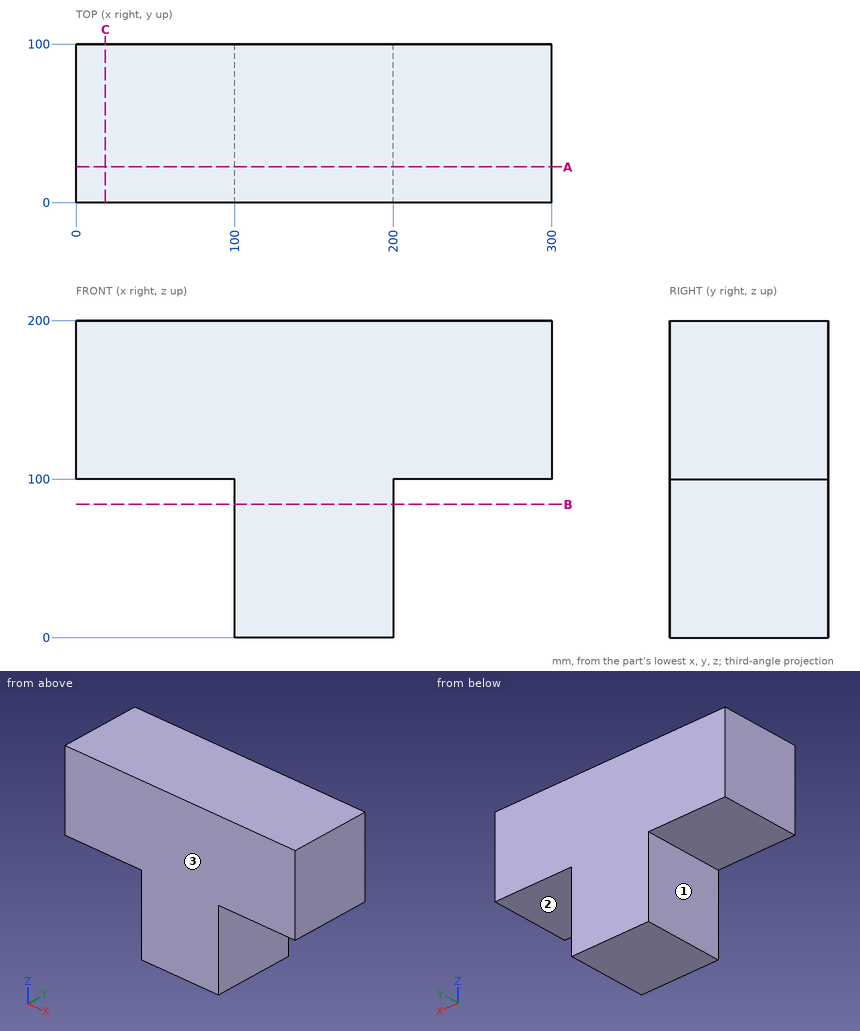
Study the drawing (mm; zero at the part's minimum x, y, z) and answer. A direction names the side the tool comes from. Give positions to 0.01 mm unless a question says otherwise; leave off trailing zeros. Order: outer loops, then holes, each group sorted by start corner. A loop starts at its lowest first (then second) coordinate and runs counter-clockwise, first axis right, second up. Notation, with made-up numbers: (-33.75, 50.25) -> (-11.75, 50.25) arc R21 ccw to (-11.75, 87.25) -> close; hole circle Ø2 at (-28.5, 19). An arc over 180 degrees is marked (long way). Put each result on its own line as item: value.
Item 1: For the marked faces 1, 2 and 3, determine the directions among +Z, -Z, +X, -X, +Y, -Y from which every point of the face is accessible in a straight line to the end or side of a thin tool.
Established:
face 1: -Z, -X, +Y, -Y
face 2: -Z, +X, +Y, -Y
face 3: +Z, -Z, +X, -X, -Y
Item 2: A straight line is drawn through the part: line 1 (Z direction, x = 80.5, y = 58.5). Find the intervals that lie inside material, in ascending order.
Established:
line 1: z = 100 to 200
Item 3: Given P1, Ø4, axis at y = 46.5, z = 130, coming from the -X side; P2, Ø1, axis at y = 37.5, z = 51, coming from the +X side; P3, Ø10, axis at x = 57.5, y = 60, coming from the -Z side, each flat-ended and moving along its own axis, determine where each tip first touches the part or whether it passes through.
Established:
P1: stops at x = 0
P2: stops at x = 200
P3: stops at z = 100
Item 4: A cutting plane is placed at A-A on y = 22.5. Give the vertices of the cut face in (x, z), plus the area to 3 significant figures.
Established:
outline: (0, 100) -> (100, 100) -> (100, 0) -> (200, 0) -> (200, 100) -> (300, 100) -> (300, 200) -> (0, 200) -> close
area: 40,000 mm^2
Item 5: A cutting plane is placed at C-C on x = 18.5. Give the vertices of the cut face in (y, z).
Established:
outline: (0, 100) -> (100, 100) -> (100, 200) -> (0, 200) -> close
Item 6: A cutting plane is placed at B-B on z = 84. Give the vertices of the cut face in (x, y).
Established:
outline: (100, 0) -> (200, 0) -> (200, 100) -> (100, 100) -> close
